```python
from build123d import *

# Parameters (mm, degrees)
BOSS_EXTRUDE3_DEPTH = 6.5
SKETCH9_R           = 2.38125
SKETCH9_R_2         = 3
SKETCH9_R_3         = 1.55
CUT_EXTRUDE4_DEPTH  = 6.5
SKETCH10_W          = 37
SKETCH10_H          = 2.5
CUT_EXTRUDE5_DEPTH  = 15
FILLET6_R           = 3
FILLET7_R           = 3
FILLET8_RADIUS      = 5
FILLET8_LENGTH      = 6.5


with BuildPart() as part:
    # Sketch8 → Boss-Extrude3 (new body)
    with BuildSketch(Plane.XY):
        with BuildLine():
            Line((-25, -5), (6.339745962, -5))
            ThreePointArc((6.339745962, -5), (25, 0), (6.339745962, 5))
            Line((6.339745962, 5), (-25, 5))
            Line((-25, 5), (-25, -5))
        make_face()
    extrude(amount=BOSS_EXTRUDE3_DEPTH)

    # Sketch9 → Cut-Extrude4 (cut)
    with BuildSketch(Plane.XY.offset(6.5)):
        with Locations((-20, 0)):
            Circle(SKETCH9_R)
        with Locations((15, 0)):
            Circle(SKETCH9_R_2)
        with Locations((22, 0)):
            Circle(SKETCH9_R_3)
        with Locations((15, -7)):
            Circle(SKETCH9_R_3)
        with Locations((8, 0)):
            Circle(SKETCH9_R_3)
        with Locations((15, 7)):
            Circle(SKETCH9_R_3)
    extrude(amount=-CUT_EXTRUDE4_DEPTH, mode=Mode.SUBTRACT)

    # Sketch10 → Cut-Extrude5 (cut, symmetric)
    with BuildSketch(Plane(origin=(0, 0, 0), x_dir=(1, 0, 0), z_dir=(0, 1, 0))):
        with Locations((6.5, -5.25)):
            Rectangle(SKETCH10_W, SKETCH10_H)
    extrude(amount=CUT_EXTRUDE5_DEPTH, both=True, mode=Mode.SUBTRACT)

    # Fillet6
    # the kernel refuses this fillet: 3 mm, written as the material it takes off along each edge
    with BuildSketch(Plane(origin=(-12, 12.395099729, 6.5), x_dir=(0, 0, -1), z_dir=(0, -1, 0))) as fillet6_piece_1:
        with BuildLine():
            CenterArc((3, -2.958039892), FILLET6_R, 99.594068227, 80.405931773)
            Line((0, -2.958039892), (-0.06, -2.958039892))
            Line((-0.06, -2.958039892), (-0.06, 0))
            Line((-0.06, 0), (0, 0.06))
            ThreePointArc((0, 0.06), (1.25, 0.06), (2.49, 0.059160798))
            Line((2.49, 0.059160798), (2.5, 0))
        make_face()
    extrude(amount=24.790199458, mode=Mode.SUBTRACT)

    # Fillet7
    fillet7_edges = [part.edges().sort_by_distance(p)[0] for p in [
        (6.339745962, -5, 2),
        (6.339745962, 5, 2),
        (-12, 0, 4),
    ]]
    fillet(fillet7_edges, radius=FILLET7_R)

    # Fillet8: full round fillet: the end face becomes a half cylinder, R = half its width
    fillet8_face = Plane((-25, 0, 3.25), x_dir=(0, 0, 1), z_dir=(-1, 0, 0))  # on the end face: x along it, z out of the body
    fillet8_slab = fillet8_face.offset(-FILLET8_RADIUS / 2) * Box(FILLET8_LENGTH, 2 * FILLET8_RADIUS, FILLET8_RADIUS, mode=Mode.PRIVATE)  # the body's end, R deep
    fillet8_round = Plane((-20, 0, 3.25), x_dir=(-1, 0, 0), z_dir=(0, 0, 1)) * Cylinder(FILLET8_RADIUS, FILLET8_LENGTH, mode=Mode.PRIVATE)  # its axis R under the face
    add(fillet8_slab - fillet8_round, mode=Mode.SUBTRACT)


solid = part.part
```
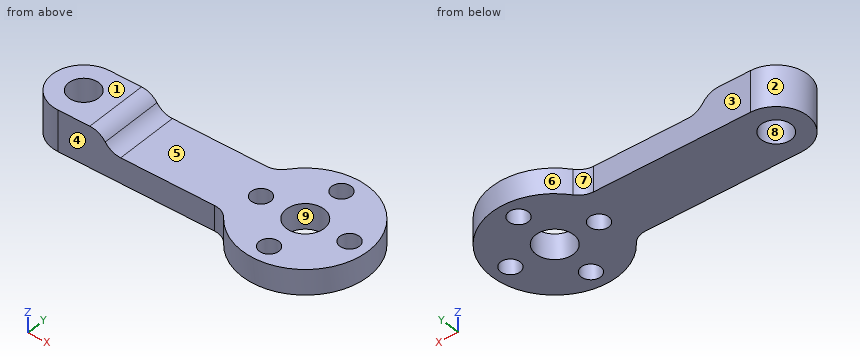
The listing builds one solid part. Answer for the finished solid, in the listing's coordinates (mm). Face numbers are marked on the shaded views. A direction names the side the tool comes from. Give positions to 0.01 mm unless a question says otherwise; leave off trailing zeros. Order: outer loops, then holes, each group sorted by start corner. A loop starts at its lowest first (then second) coordinate and runs counter-clockwise, first axis right, second up. Notation, with made-up numbers: (-31, 51) -> (-8, 51) arc R20 cw to (-8, 71) -> close; hole circle Ø4 at (68.5, 53). An arc over 180 degrees is marked (long way). Write each question's results on one line, items separated by ' | '.
Q1. The part is cut by section A-A, the plane x = 15. Give the vertices of the cut face in (y, z).
Checked values:
outline: (-10, 0) -> (-8.55, 0) -> (-8.55, 4) -> (-10, 4) -> close; (-5.45, 0) -> (-3, 0) -> (-3, 4) -> (-5.45, 4) -> close; (3, 0) -> (5.45, 0) -> (5.45, 4) -> (3, 4) -> close; (8.55, 0) -> (10, 0) -> (10, 4) -> (8.55, 4) -> close
Q2. Each of these flat-tipped pins is pushed along its axis until it touches: P1, Ø3, axis at x = 18.5, z = 5, coming from the -Y side; P2, Ø4, axis at x = 8, y = 0, coming from the +Z side; P3, Ø2, axis at x = -6.5, z = 4, coming from the +Y side. Where does it stop, or does it pass through?
Checked values:
P1: stops at y = -9.71 | P2: stops at z = 4 | P3: stops at y = 5
Q3. Which of the six approach directions +Z, -Z, +X, -X, +Y, -Y give full straight-line access (tool end or side, diameter ignored) to the marked faces 1, 2, 3, 4 and 5?
Checked values:
face 1: +Z, +X, -X, +Y, -Y | face 2: +Z, -Z, -X | face 3: +Z, -Z, -X, +Y | face 4: +Z, -Z, -X, -Y | face 5: +Z, +X, +Y, -Y
Q4. Determine the mould class of the marked faces 6, 7, 8 and 9 for opening direction Y: pulls with the +Y half, pulls with the -Y half, needs draft (parallel to the pull), parting line crosses it, or undercut.
Checked values:
face 6: parting line crosses it | face 7: pulls with the +Y half | face 8: undercut | face 9: undercut
Q5. The part is cut by section C-C, the plane z = 3. Give the vertices of the cut face in (x, y).
Checked values:
outline: (-20, -5) -> (4.75, -5) arc R3 cw to (7.12, -6.15) arc R10 ccw (long way) to (7.12, 6.15) arc R3 cw to (4.75, 5) -> (-20, 5) arc R5 ccw to start; hole circle Ø4.76 at (-20, 0); hole circle Ø3.1 at (8, 0); hole circle Ø6 at (15, 0); hole circle Ø3.1 at (15, -7); hole circle Ø3.1 at (15, 7); hole circle Ø3.1 at (22, 0)
Q6. Straight lines are drawn through the part: probe 1 along Y at (x, z) = (15, 1.3); probe 2 along Y at (x, z) = (4, 3.75); probe 3 along Y at (x, z) = (8, 2.75). For each, find the intervals that lie inside material, in ascending order. Write a range as from..to.
Checked values:
probe 1: y = -10..-8.55, -5.45..-3, 3..5.45, 8.55..10 | probe 2: y = -5..5 | probe 3: y = -7.14..-1.55, 1.55..7.14
Q7. The part is cut by section B-B, the plane y = 0. Give the vertices of the cut face in (x, z).
Checked values:
outline: (-25, 0) -> (-22.38, 0) -> (-22.38, 6.5) -> (-25, 6.5) -> close; (-17.62, 0) -> (6.45, 0) -> (6.45, 4) -> (-10.08, 4) arc R3 cw to (-12.52, 5.25) arc R3 ccw to (-14.96, 6.5) -> (-17.62, 6.5) -> close; (9.55, 0) -> (12, 0) -> (12, 4) -> (9.55, 4) -> close; (18, 0) -> (20.45, 0) -> (20.45, 4) -> (18, 4) -> close; (23.55, 0) -> (25, 0) -> (25, 4) -> (23.55, 4) -> close
Q8. The part is cut by section D-D, the plane x = 8. Give the vertices of the cut face in (y, z).
Checked values:
outline: (-7.14, 0) -> (-1.55, 0) -> (-1.55, 4) -> (-7.14, 4) -> close; (1.55, 0) -> (7.14, 0) -> (7.14, 4) -> (1.55, 4) -> close
